from build123d import *

# Parameters (mm, degrees)
SKETCH1_R           = 9.5
BOSS_EXTRUDE1_DEPTH = 12
SKETCH4_R           = 19
SKETCH4_R_2         = 2
BOSS_EXTRUDE3_DEPTH = 3.8
CUT_EXTRUDE2_DEPTH  = 20
SKETCH5_R           = 1.5
CUT_EXTRUDE3_DEPTH  = 5


with BuildPart() as part:
    # Sketch1 → Boss-Extrude1 (new body)
    with BuildSketch(Plane(origin=(0, 0, 0), x_dir=(0, 0, -1), z_dir=(1, 0, 0))):
        Circle(SKETCH1_R)
    extrude(amount=BOSS_EXTRUDE1_DEPTH)

    # Sketch4 → Boss-Extrude3 (add)
    with BuildSketch(Plane.ZY):
        Circle(SKETCH4_R)
        with Locations((-10.5, 10.5)):
            Circle(SKETCH4_R_2, mode=Mode.SUBTRACT)
        with Locations((10.5, 10.5)):
            Circle(SKETCH4_R_2, mode=Mode.SUBTRACT)
        with Locations((10.5, -10.5)):
            Circle(SKETCH4_R_2, mode=Mode.SUBTRACT)
        with Locations((-10.5, -10.5)):
            Circle(SKETCH4_R_2, mode=Mode.SUBTRACT)
    extrude(amount=BOSS_EXTRUDE3_DEPTH)

    # Sketch2 → Cut-Extrude2 (cut)
    with BuildSketch(Plane(origin=(12, 0, 0), x_dir=(0, 0, -1), z_dir=(1, 0, 0))):
        with BuildLine():
            Line((-1.5, 6.319696007), (1.5, 6.319696007))
            Line((1.5, 6.319696007), (1.5, 4.91426495))
            ThreePointArc((1.5, 4.91426495), (1.537093703, 4.79824108), (1.634615385, 4.72525476))
            ThreePointArc((1.634615385, 4.72525476), (0, -5), (-1.634615385, 4.72525476))
            ThreePointArc((-1.634615385, 4.72525476), (-1.537093703, 4.79824108), (-1.5, 4.91426495))
            Line((-1.5, 4.91426495), (-1.5, 6.319696007))
        make_face()
    extrude(amount=-CUT_EXTRUDE2_DEPTH, mode=Mode.SUBTRACT)

    # Sketch5 → Cut-Extrude3 (cut)
    with BuildSketch(Plane.XZ.offset(-6.319696007)):
        with Locations((6, 0)):
            Circle(SKETCH5_R)
    extrude(amount=-CUT_EXTRUDE3_DEPTH, mode=Mode.SUBTRACT)


solid = part.part
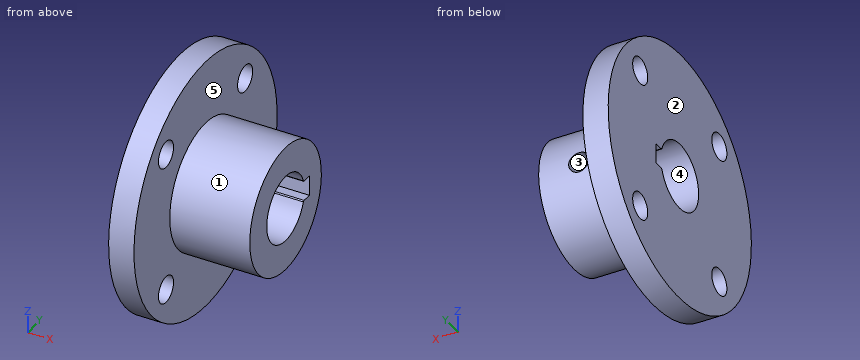
For this review, take the finished solid that the model builds, in its own axes (mm). Face numbers are marked on the shaded views. A direction names the side the tool comes from. Give positions to 0.01 mm unless a question says otherwise; leave off trailing zeros. Order: outer loops, then holes, each group sorted by start corner. A loop starts at its lowest first (then second) coordinate and runs counter-clockwise, first axis right, second up. Notation, with made-up numbers: (-25.75, 39.25) -> (11.25, 39.25) arc R13 cw to (11.25, 43.25) -> close; hole circle Ø11 at (62.25, 81.5). An arc over 180 degrees is marked (long way). Write item = value, one per line.
1) We need section C-C, the plane z = 0. Give the boundary of the cut face in (x, y).
Findings:
outline = (-3.8, -19) -> (0, -19) -> (0, -9.5) -> (12, -9.5) -> (12, -5) -> (-3.8, -5) -> close; (-3.8, 6.32) -> (4.5, 6.32) -> (4.5, 9.5) -> (0, 9.5) -> (0, 19) -> (-3.8, 19) -> close; (7.5, 6.32) -> (12, 6.32) -> (12, 9.5) -> (7.5, 9.5) -> close
2) For the marked faces 1 and 2, list the 3-axis set-ups (+Z, -Z, +X, -X, +Y, -Y) from which the entire face can be reached by the end or side of a thin tool; tool diameter is ignored.
Findings:
face_1 = +X
face_2 = +Z, -Z, -X, +Y, -Y
3) To check wall thickness, follow L1, parallel to Z at x = -1.5, y = -10; L2, parallel to Y at x = -1.2, z = -10.5; L3, parallel to Y at x = 8, z = -4. State the ranges of each line that lie inside material, in increasing order. Write a range as from..to.
Findings:
L1 = -16.16..-12.44, -8.56..8.56, 12.44..16.16
L2 = -15.84..-12.5, -8.5..8.5, 12.5..15.84
L3 = -8.62..-3, 3..8.62
4) We need section A-A, the plane x = -1. Give the boundary of the cut face in (y, z), and give its area (3 significant figures).
Findings:
outline = circle Ø38 at (0, 0); hole circle Ø4 at (-10.5, -10.5); hole circle Ø4 at (-10.5, 10.5); hole (4.73, -1.63) arc R0.2 cw to (4.91, -1.5) -> (6.32, -1.5) -> (6.32, 1.5) -> (4.91, 1.5) arc R0.2 cw to (4.73, 1.63) arc R5 ccw (long way) to start; hole circle Ø4 at (10.5, -10.5); hole circle Ø4 at (10.5, 10.5)
area = 1,000 mm^2
5) Draft analysis for pull direction X (two halves, no side actions). For the marked faces 3, 4 and 5, state which applies: pulls with the +X half, pulls with the -X half, needs draft (parallel to the pull), parting line crosses it, or undercut.
Findings:
face_3 = undercut
face_4 = needs draft
face_5 = pulls with the +X half
6) We need section D-D, the plane y = 10. Give the boundary of the cut face in (x, z).
Findings:
outline = (-3.8, -16.16) -> (0, -16.16) -> (0, -12.44) -> (-3.8, -12.44) -> close; (-3.8, -8.56) -> (0, -8.56) -> (0, 8.56) -> (-3.8, 8.56) -> close; (-3.8, 12.44) -> (0, 12.44) -> (0, 16.16) -> (-3.8, 16.16) -> close
7) We need section B-B, the plane y = 0. Give the boundary of the cut face in (x, z), and give its area (3 significant figures).
Findings:
outline = (-3.8, -19) -> (0, -19) -> (0, -9.5) -> (12, -9.5) -> (12, -5) -> (-3.8, -5) -> close; (-3.8, 5) -> (12, 5) -> (12, 9.5) -> (0, 9.5) -> (0, 19) -> (-3.8, 19) -> close
area = 214 mm^2
8) Insertion check: pin 1 (12 mm diameter, centred on y = 15, z = -7.5, fed in from +X); pin 2 (2.5 mm diameter, centred on x = 0.5, z = 0, fed in from -Y); pin 3 (1.5 mm diameter, centred on x = 7, y = 5.5, fed in from +Z); pin 4 (5 mm diameter, centred on x = 5.5, z = -12.5, fed in from -Y). Each pin has a flat end and moves straight along its axis. Give the tip position at first contact, or say it passes through.
Findings:
pin_1 = 0
pin_2 = -19
pin_3 = 8.23
pin_4 = through
